Geometry check sheet. Reference: the model listing, model coordinates, mm. A direction names the side the tool comes from. Give positions to 0.01 mm unless a question says otherwise; leave off trailing zeros. Write each loop counter-clockwise with the first axis right and the second up, starting at its lowest first coordinate (ties: lowest second). Pieces come first, ordered by that corner, then holes.
(1) Depth check by flat-ended pin: P1, Ø1, axis at x = 41, y = 1, coming from the +Z side (3 decimals); P2, Ø1.5, axis at x = 7, y = 0.5, coming from the -Z side; P3, Ø1, axis at y = 1, z = -14, coming from the -X side; P4, Ø4.5, axis at x = 134.93, z = 14.2, coming from the +Y side. Enter the tip coordinate at first touch or a pass-through.
(2) Thickness scan on line 1 along Z through (x, y) = (-2, 2.8); line 2 along Z through (x, y) = (71.5, 2); line 3 along X through (y, z) = (0.6, 0.5). Record the ranges inside material, lowest first.
(3) Tool access check on faces 4 (the flat face through (154.235, 1.565, -28.084)), 5 (the flat face through (68.591, 1.61, 8.664)). Record the directions out of +Z, -Z, +X, -X, +Y, -Y that give a thin tool (end or side, any length) a straight path to the whole face; none if there is none.
(4) Cross-section at A-A (z = -37). Record the boundary of the cut face in (x, y) (3 decimals).
(5) Cross-section at C-C (x = 73). Record the boundary of the cut face in (y, z) (3 decimals).
(6) Mould release check, pull along X, two halves, no side actions. Record for faces 1 (the cylindrical face through (139.826, 1.565, 19.549)), 2 (the cylindrical face through (-3.61, 1.565, -61.318)), 3 (the flat face through (78.553, 1.565, -74.508)): +X half, -X half, draft (parallel to the pull), parting line (faces both ways), or undercut.
(7) Cross-section at B-B (y = 2.2). Count the separate pieces of the cut face and the enclosed holes in it, and give its area (3 significant figures).
(8) Cross-section at D-D (x = 101.5). Record the boundary of the cut face in (y, z) (3 decimals).
```python
from build123d import *

# Parameters (mm, degrees)
SKETCH1_R            = 2.4892
BOSS_EXTRUDE1_DEPTH  = 3.175
TRIGGER_CUTOUT_DEPTH = 3.175
SERVO_CUTOUT_DEPTH   = 3.175


with BuildPart() as part:
    # Sketch1 → Boss-Extrude1 (new body)
    with BuildSketch(Plane(origin=(0, 0, 0), x_dir=(1, 0, 0), z_dir=(0, 1, 0))):
        with BuildLine():
            Line((-6.8229868, -7.488197853), (47.14701474, -37.472309865))
            ThreePointArc((47.14701474, -37.472309865), (49.553689318, -38.298669515), (52.097667916, -38.242761734))
            Line((52.097667916, -38.242761734), (136.359344262, -21.308190288))
            ThreePointArc((136.359344262, -21.308190288), (139.866879533, -19.510833837), (141.916296901, -16.144354617))
            Line((141.916296901, -16.144354617), (166.90343399, 73.568749369))
            ThreePointArc((166.90343399, 73.568749369), (165.462253091, 80.188248266), (159.182077212, 82.728751949))
            Line((159.182077212, 82.728751949), (-4.366145722, 66.053653766))
            ThreePointArc((-4.366145722, 66.053653766), (-9.125920254, 63.663982971), (-10.969503308, 58.667265887))
            Line((-10.969503308, 58.667265887), (-10.288924124, -1.672992978))
            ThreePointArc((-10.288924124, -1.672992978), (-9.33910622, -5.047363397), (-6.8229868, -7.488197853))
        make_face()
        with Locations(Location((159.917634832, 75.514453101, 0), (0, 0, 270))):
            Circle(SKETCH1_R, mode=Mode.SUBTRACT)
        with Locations(Location((134.930497743, -14.198650885, 0), (0, 0, 270))):
            Circle(SKETCH1_R, mode=Mode.SUBTRACT)
        with Locations(Location((50.668821397, -31.133222331, 0), (0, 0, 270))):
            Circle(SKETCH1_R, mode=Mode.SUBTRACT)
        with Locations(Location((-3.719648143, 58.830829265, 0), (0, 0, 270))):
            Circle(SKETCH1_R, mode=Mode.SUBTRACT)
        with Locations(Location((-3.508126319, -0.086017173, 0), (0, 0, 270))):
            Circle(SKETCH1_R, mode=Mode.SUBTRACT)
    extrude(amount=BOSS_EXTRUDE1_DEPTH)

    # Sketch3 → trigger cutout (cut)
    with BuildSketch(Plane(origin=(0, 3.175, 0), x_dir=(1, 0, 0), z_dir=(0, 1, 0))):
        Polygon((41.255934536, -15.678441329), (66.468104622, -13.883980824), (70.774809833, -3.296663849), (70.032795293, 7.128640439), (58.56546888, 6.312460623), (53.862019579, 3.583115238), (41.255934536, 0), align=None)
    extrude(amount=-TRIGGER_CUTOUT_DEPTH, mode=Mode.SUBTRACT)

    # Sketch4 → servo cutout (cut)
    with BuildSketch(Plane(origin=(0, 3.175, 0), x_dir=(1, 0, 0), z_dir=(0, 1, 0))):
        Polygon((44.328297275, 43.5580507), (84.328297275, 43.5580507), (84.328297275, 15.7580507), (91.578297275, 15.7580507), (91.578297275, 11.409751948), (84.328297275, 11.409751948), (84.328297275, 3.0580507), (64.328297275, 3.0580507), (64.328297275, -2.168421287), (44.328297275, -2.168421287), (44.328297275, 3.0580507), (44.328297275, 11.409751948), (37.078297275, 11.409751948), (37.078297275, 15.7580507), (44.328297275, 15.7580507), align=None)
    extrude(amount=-SERVO_CUTOUT_DEPTH, mode=Mode.SUBTRACT)


solid = part.part
```
Reply:
1. P1: stops at z = 34.335
1. P2: stops at z = -67.29
1. P3: stops at x = -10.47
1. P4: passes through
2. line 1: z = -66.29 to -60.63, -57.03 to -1.89, 2.07 to 10.17
2. line 2: z = -73.79 to -43.56, -3.06 to 34.34
2. line 3: x = -10.3 to -5.96, -1.05 to 41.26, 70.58 to 146.27
3. face 4: +Z, +X, +Y, -Y
3. face 5: +Y, -Y
4. outline: (-10.725, 0) - (44.328, 0) - (44.328, 3.175) - (-10.725, 3.175) - close; (84.328, 0) - (156.718, 0) - (156.718, 3.175) - (84.328, 3.175) - close
5. outline: (0, -73.942) - (3.175, -73.942) - (3.175, -43.558) - (0, -43.558) - close; (0, -3.058) - (3.175, -3.058) - (3.175, 34.042) - (0, 34.042) - close
6. face 1: +X half
6. face 2: undercut
6. face 3: -X half
7. separate pieces: 1
7. enclosed holes: 6
7. area: 14,300 mm2
8. outline: (0, -76.848) - (3.175, -76.848) - (3.175, 28.314) - (0, 28.314) - close
